Can you work these out from the drawing? Everything is in mm from the part's minimum corner. A direction names the side the tool comes from. Coordinates: 2 decimals unless noted, no trailing zeros. Order: outer loops, then holes, each group sorted by start corner. A loop starts at its lowest first (then second) coordinate and runs counter-clockwise, first axis right, second up. Notation, with made-up numbers: (69, 72) -> (119, 72) arc R30 ccw to (119, 111) -> close; hole circle Ø3 at (7, 50). An arc over 180 degrees is marked (long way). Answer in a Markdown table with one row per item.
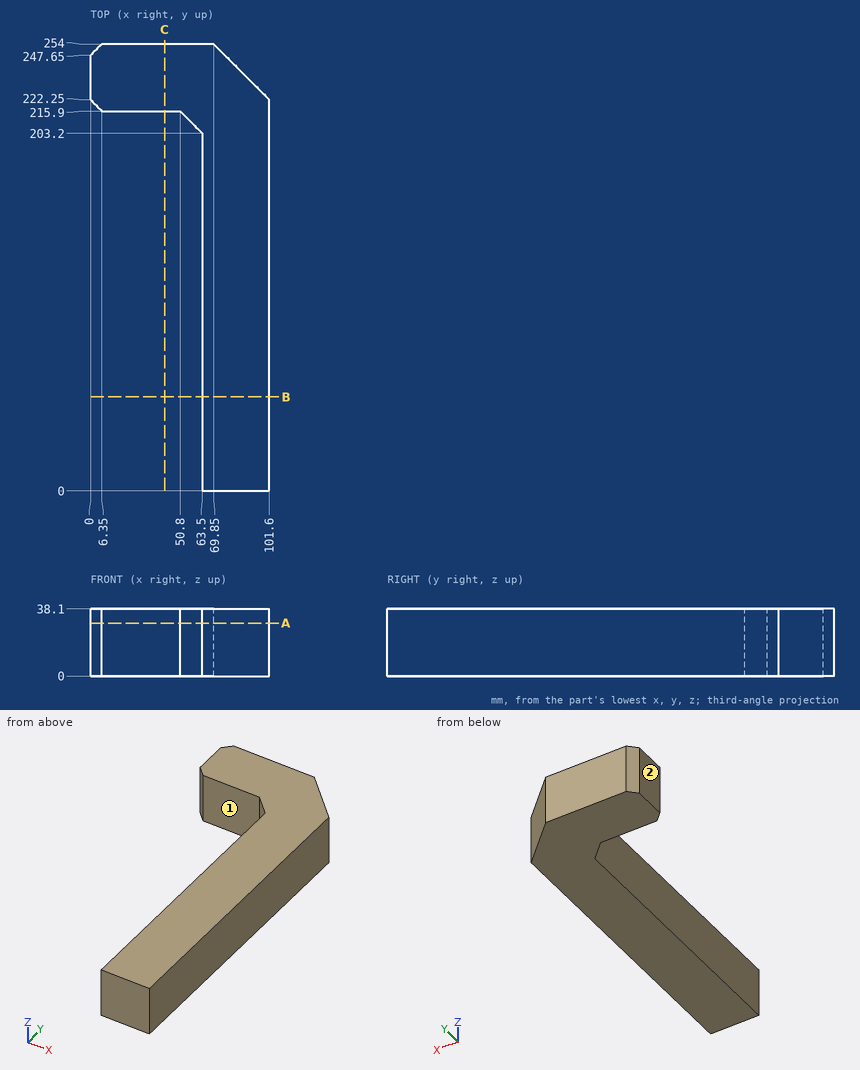
(1) On a 3-axis mill with a long thin cutter (end or side, diameter ignored), from which of +Z, -Z, +X, -X, +Y, -Y can I reach the whole of each face in a straight line? I mean the marked faces 1 and 2. Say none if no direction works.
Response values:
| item | result |
|---|---|
| face 1 | +Z, -Z, -X, -Y |
| face 2 | +Z, -Z, -X, +Y, -Y |
(2) I need wall thicknesses on line 1 (Y direction, x = 48, z = 17); line 2 (X direction, y = 199, z = 25.5); line 3 (X direction, y = 242, z = 25). Which ranges of each line are inside material? Lowest first, please. Write a range as [from, to].
Response values:
| item | result |
|---|---|
| line 1 | [215.9, 254] |
| line 2 | [63.5, 101.6] |
| line 3 | [0, 81.85] |
(3) Suppose I cut it at C-C (x = 42). Please give me the cut outline in (y, z).
Response values:
| item | result |
|---|---|
| outline | (215.9, 0) -> (254, 0) -> (254, 38.1) -> (215.9, 38.1) -> close |
(4) Suppose I cut it at A-A (z = 30). Please give me the cut outline in (x, y), and give its area (3 significant figures).
Response values:
| item | result |
|---|---|
| outline | (0, 222.25) -> (6.35, 215.9) -> (50.8, 215.9) -> (63.5, 203.2) -> (63.5, 0) -> (101.6, 0) -> (101.6, 222.25) -> (69.85, 254) -> (6.35, 254) -> (0, 247.65) -> close |
| area | 11,600 mm2 |
(5) Will these pins go through, and if not, where does the flat tip stop? pin 1 Ø11.5 at (y, z) = (63, 17.5) entering from -X; pin 2 Ø6 at (x, z) = (66.5, 25.5) entering from -Y; pin 3 Ø1.5 at (x, z) = (34, 26.5) entering from -Y.
Response values:
| item | result |
|---|---|
| pin 1 | x = 63.5 |
| pin 2 | y = 0 |
| pin 3 | y = 215.9 |
(6) Suppose I cut it at B-B (y = 53.5). Please give me the cut outline in (x, z).
Response values:
| item | result |
|---|---|
| outline | (63.5, 0) -> (101.6, 0) -> (101.6, 38.1) -> (63.5, 38.1) -> close |
